from build123d import *

# Parameters (mm, degrees)
SKETCH1_W            = 208
SKETCH1_H            = 147
BOSS_EXTRUDE1_DEPTH  = 1
CUT_EXTRUDE1_DEPTH   = 128.354819304
MIRROR2_COPY_1_DEPTH = 128.354819304
FILLET1_R            = 10
CUT_EXTRUDE2_DEPTH   = 128.354819304
BOSS_EXTRUDE2_DEPTH  = 20
FILLET2_R            = 5
FILLET2_OF_MIRROR3_R = 5
MIRROR4_START        = 1
MIRROR4_DEPTH        = 20
SKETCH7_R            = 4
BOSS_EXTRUDE3_DEPTH  = 45
SKETCH8_R            = 3
CUT_EXTRUDE4_DEPTH   = 30


# Read off the part's stored shape, not the designer's step: Mirror4
with BuildPart() as part:
    # Sketch1 → Boss-Extrude1 (new body)
    with BuildSketch(Plane(origin=(0, 0, 0), x_dir=(1, 0, 0), z_dir=(0, 1, 0))):
        Rectangle(SKETCH1_W, SKETCH1_H)
    extrude(amount=BOSS_EXTRUDE1_DEPTH)

    # Sketch3 → Cut-Extrude1 (cut, through all)
    with BuildSketch(Plane(origin=(0, 1, 0), x_dir=(1, 0, 0), z_dir=(0, 1, 0))):
        with BuildLine():
            Line((-89, 83.145473262), (-89, 63.145473262))
            Line((-89, 63.145473262), (-44, 63.145473262))
            Line((-44, 63.145473262), (-44, 58.145473262))
            Line((-44, 58.145473262), (-29, 58.145473262))
            Line((-29, 58.145473262), (-29, 63.145473262))
            Line((-29, 63.145473262), (-14, 63.145473262))
            ThreePointArc((-14, 63.145473262), (-6.928932188, 63.647998579), (0, 65.145473262))
            Line((0, 65.145473262), (0, 85.145473262))
            Line((0, 85.145473262), (-89, 85.145473262))
            Line((-89, 85.145473262), (-89, 83.145473262))
        make_face()
    cut_extrude1 = extrude(amount=-CUT_EXTRUDE1_DEPTH, mode=Mode.SUBTRACT)

    # Mirror1: Cut-Extrude1 across plane
    add(cut_extrude1.mirror(Plane.XY), mode=Mode.SUBTRACT)

    # Mirror2: Cut-Extrude1 across plane
    add(cut_extrude1.mirror(Plane(origin=(0, 0, 0), x_dir=(0, 0, 1), z_dir=(1, 0, 0))), mode=Mode.SUBTRACT)

    # Mirror2 copy 1 sketch → Mirror2 copy 1 (cut, through all)
    with BuildSketch(Plane(origin=(0, 1, 0), x_dir=(-1, 0, 0), z_dir=(0, 1, 0))):
        with BuildLine():
            Line((-89, 83.145473262), (-89, 63.145473262))
            Line((-89, 63.145473262), (-44, 63.145473262))
            Line((-44, 63.145473262), (-44, 58.145473262))
            Line((-44, 58.145473262), (-29, 58.145473262))
            Line((-29, 58.145473262), (-29, 63.145473262))
            Line((-29, 63.145473262), (-14, 63.145473262))
            ThreePointArc((-14, 63.145473262), (-6.928932188, 63.647998579), (0, 65.145473262))
            Line((0, 65.145473262), (0, 85.145473262))
            Line((0, 85.145473262), (-89, 85.145473262))
            Line((-89, 85.145473262), (-89, 83.145473262))
        make_face()
    extrude(amount=-MIRROR2_COPY_1_DEPTH, mode=Mode.SUBTRACT)

    # Fillet1
    fillet1_edges = [part.edges().sort_by_distance(p)[0] for p in [
        (104, 0.5, 73.5),
        (-104, 0.5, 73.5),
        (-104, 0.5, -73.5),
        (104, 0.5, -73.5),
    ]]
    fillet(fillet1_edges, radius=FILLET1_R)

    # Sketch4 → Cut-Extrude2 (cut, through all)
    with BuildSketch(Plane.XZ):
        with BuildLine():
            Line((-58.225796132, 1.876244538), (-49.924870206, 1.876244538))
            ThreePointArc((-49.924870206, 1.876244538), (-49.217763425, 1.583351319), (-48.924870206, 0.876244538))
            Line((-48.924870206, 0.876244538), (-48.924870206, -0.876244538))
            ThreePointArc((-48.924870206, -0.876244538), (-49.217763425, -1.583351319), (-49.924870206, -1.876244538))
            Line((-49.924870206, -1.876244538), (-58.225796132, -1.876244538))
            ThreePointArc((-58.225796132, -1.876244538), (-58.932902913, -2.169137757), (-59.225796132, -2.876244538))
            Line((-59.225796132, -2.876244538), (-59.225796132, -11.176244538))
            ThreePointArc((-59.225796132, -11.176244538), (-59.518689351, -11.883351319), (-60.225796132, -12.176244538))
            Line((-60.225796132, -12.176244538), (-62.62394428, -12.176244538))
            ThreePointArc((-62.62394428, -12.176244538), (-63.331051061, -11.883351319), (-63.62394428, -11.176244538))
            Line((-63.62394428, -11.176244538), (-63.62394428, -2.876244538))
            ThreePointArc((-63.62394428, -2.876244538), (-63.916837499, -2.169137757), (-64.62394428, -1.876244538))
            Line((-64.62394428, -1.876244538), (-72.924870206, -1.876244538))
            ThreePointArc((-72.924870206, -1.876244538), (-73.631976987, -1.583351319), (-73.924870206, -0.876244538))
            Line((-73.924870206, -0.876244538), (-73.924870206, 0.876244538))
            ThreePointArc((-73.924870206, 0.876244538), (-73.631976987, 1.583351319), (-72.924870206, 1.876244538))
            Line((-72.924870206, 1.876244538), (-64.62394428, 1.876244538))
            ThreePointArc((-64.62394428, 1.876244538), (-63.916837499, 2.169137757), (-63.62394428, 2.876244538))
            Line((-63.62394428, 2.876244538), (-63.62394428, 11.823755462))
            ThreePointArc((-63.62394428, 11.823755462), (-63.331051061, 12.530862243), (-62.62394428, 12.823755462))
            Line((-62.62394428, 12.823755462), (-60.225796132, 12.823755462))
            ThreePointArc((-60.225796132, 12.823755462), (-59.518689351, 12.530862243), (-59.225796132, 11.823755462))
            Line((-59.225796132, 11.823755462), (-59.225796132, 2.876244538))
            ThreePointArc((-59.225796132, 2.876244538), (-58.932902913, 2.169137757), (-58.225796132, 1.876244538))
        make_face()
    extrude(amount=-CUT_EXTRUDE2_DEPTH, mode=Mode.SUBTRACT)

    # Sketch5 → Boss-Extrude2 (add)
    with BuildSketch(Plane(origin=(0, 1, 0), x_dir=(1, 0, 0), z_dir=(0, 1, 0))):
        Polygon((-104, 36.429300806), (-11, 36.429300806), (-11, 63.235554408), (-14, 63.145473262), (-14, 39.429300806), (-104, 39.429300806), align=None)
    boss_extrude2 = extrude(amount=BOSS_EXTRUDE2_DEPTH)

    # Fillet2
    fillet2_edges = [part.edges().sort_by_distance(p)[0] for p in [
        (-11, 11, -36.429300806),
    ]]
    fillet(fillet2_edges, radius=FILLET2_R)

    # Mirror3: Boss-Extrude2 across plane
    add(boss_extrude2.mirror(Plane.XY))

    # Fillet2 of Mirror3
    fillet2_of_mirror3_edges = [part.edges().sort_by_distance(p)[0] for p in [
        (-11, 11, 36.429300806),
    ]]
    fillet(fillet2_of_mirror3_edges, radius=FILLET2_OF_MIRROR3_R)

    # Mirror4 outline → Mirror4 (add)
    with BuildSketch(Plane(origin=(0, 0, 0), x_dir=(1, 0, 0), z_dir=(0, 1, 0)).offset(MIRROR4_START)):
        with BuildLine():
            Line((104, -39.429300806), (104, -36.429300806))
            Line((104, -36.429300806), (16, -36.429300806))
            ThreePointArc((16, -36.429300806), (12.464466094, -37.8937669), (11, -41.429300806))
            Line((11, -41.429300806), (11, -63.235554408))
            Line((11, -63.235554408), (14, -63.145473262))
            Line((14, -63.145473262), (14, -39.429300806))
            Line((14, -39.429300806), (104, -39.429300806))
        make_face()
        with BuildLine():
            Line((104, 36.429300806), (104, 39.429300806))
            Line((104, 39.429300806), (14, 39.429300806))
            Line((14, 39.429300806), (14, 63.145473262))
            Line((14, 63.145473262), (11, 63.235554408))
            Line((11, 63.235554408), (11, 41.429300806))
            ThreePointArc((11, 41.429300806), (12.464466094, 37.8937669), (16, 36.429300806))
            Line((16, 36.429300806), (104, 36.429300806))
        make_face()
    extrude(amount=MIRROR4_DEPTH)

    # Sketch7 → Boss-Extrude3 (add)
    with BuildSketch(Plane.XZ):
        with Locations(Location((97, 65, 0), (0, 0, 90))):
            Circle(SKETCH7_R)
        with Locations(Location((-95, 65, 0), (0, 0, 90))):
            Circle(SKETCH7_R)
        with Locations(Location((-95, -65, 0), (0, 0, 90))):
            Circle(SKETCH7_R)
        with Locations(Location((97, -65, 0), (0, 0, 90))):
            Circle(SKETCH7_R)
    extrude(amount=BOSS_EXTRUDE3_DEPTH)

    # Sketch8 → Cut-Extrude4 (cut)
    with BuildSketch(Plane(origin=(0, -45, 0), x_dir=(-1, 0, 0), z_dir=(0, -1, 0))):
        with Locations(Location((95, 65, 0), (0, 0, 90))):
            Circle(SKETCH8_R)
        with Locations(Location((95, -65, 0), (0, 0, 90))):
            Circle(SKETCH8_R)
        with Locations(Location((-97, -65, 0), (0, 0, 90))):
            Circle(SKETCH8_R)
        with Locations(Location((-97, 65, 0), (0, 0, 90))):
            Circle(SKETCH8_R)
    extrude(amount=-CUT_EXTRUDE4_DEPTH, mode=Mode.SUBTRACT)


solid = part.part
Could you check a few things on this model? Use its own coordinates, in mm. A direction names the side the tool comes from. Coordinates: 2 decimals unless noted, no trailing zeros. Order: outer loops, then holes, each group sorted by start corner. A loop starts at its lowest first (then second) coordinate and runs counter-clockwise, first axis right, second up. Notation, with made-up numbers: (70.25, 26.5) -> (82.25, 26.5) arc R15 cw to (82.25, 36.5) -> close; hole circle Ø9 at (-7, 54.25). An arc over 180 degrees is marked (long way). One line per item, written item: value. Start each with the question number.
1) We'd pull the mould along Z, two halves only. Please class faces 1 (the flat face through (58, 1, 52)), 2 (the cylindrical face through (101.15, 0.51, 70.49)), 3 (the flat face through (-95, -15, -65)): +Z half, -Z half, draft (parallel to the pull), parting line (faces both ways), or undercut.
2) Imagine slicing it at B-B on z = -9. List the corners of the cut face in (x, y) for me, plus the area to 3 significant figures.
3) If I drill on L1, parallel to X at y = -31, z = -65; L2, parallel to Z at x = 40, y = 17; L3, parallel to Y at x = -50, z = 53, over which ranges is the centre line in solid material (lowest first)? Write a range as [from, to].
4) Imagine slicing it at D-D on x = 57. List the corners of the cut face in (y, z) for me, plus the area to 3 significant figures.
5) Which directions (+Z, -Z, +X, -X, +Y, -Y) give clear straight access to the entire face, cutting with the end or side of a thin tool? Please do faces 4 (the flat face through (-60, 1, 52)), 5 (the flat face through (-58, 11, -39.429)), 6 (the cylindrical face through (94.07, -30.21, -64.35)), 7 (the flat face through (-11, 11, -52)).
6) Imagine slicing it at A-A on y = -19.5. List the corners of the cut face in (x, z) for me, plus the area to 3 significant figures.
7) I'm going to push flat-ended pins straight in: pin 1 (3.5 mm diameter, centred on x = -95, z = 65, fed in from +Y); pin 2 (6 mm diameter, centred on x = 4.5, z = 18, fed in from -Y); pin 3 (1.1 mm diameter, centred on x = 22.5, y = 0.5, fed in from -Z). Where does each tip first touch, or does it pass through?
8) Imagine slicing it at C-C on y = 15. List the corners of the cut face in (x, z) for me, plus the area to 3 significant figures.
Answer list:
1. face 1: draft
1. face 2: +Z half
1. face 3: undercut
2. outline: (-104, 0) -> (-63.62, 0) -> (-63.62, 1) -> (-104, 1) -> close; (-59.23, 0) -> (104, 0) -> (104, 1) -> (-59.23, 1) -> close
2. area: 204 mm2
3. L1: x = [-99, -98], [-92, -91], [93, 94], [100, 101]
3. L2: z = [-39.43, -36.43], [36.43, 39.43]
3. L3: y = [0, 1]
4. outline: (0, -63.15) -> (1, -63.15) -> (1, -39.43) -> (21, -39.43) -> (21, -36.43) -> (1, -36.43) -> (1, 36.43) -> (21, 36.43) -> (21, 39.43) -> (1, 39.43) -> (1, 63.15) -> (0, 63.15) -> close
4. area: 246 mm2
5. face 4: +Z, -X, +Y
5. face 5: -Z, -X, +Y
5. face 6: -Y
5. face 7: +Z, -Z, +Y
6. outline: circle Ø8 at (-95, -65); circle Ø8 at (-95, 65); circle Ø8 at (97, -65); circle Ø8 at (97, 65); hole circle Ø6 at (-95, -65); hole circle Ø6 at (-95, 65); hole circle Ø6 at (97, -65); hole circle Ø6 at (97, 65)
6. area: 88.0 mm2
7. pin 1: stops at y = 1
7. pin 2: stops at y = 0
7. pin 3: stops at z = -63.15
8. outline: (-104, -39.43) -> (-14, -39.43) -> (-14, -63.15) -> (-11, -63.24) -> (-11, -41.43) arc R5 ccw to (-16, -36.43) -> (-104, -36.43) -> close; (-104, 36.43) -> (-16, 36.43) arc R5 ccw to (-11, 41.43) -> (-11, 63.24) -> (-14, 63.15) -> (-14, 39.43) -> (-104, 39.43) -> close; (11, -63.24) -> (14, -63.15) -> (14, -39.43) -> (104, -39.43) -> (104, -36.43) -> (16, -36.43) arc R5 ccw to (11, -41.43) -> close; (11, 41.43) arc R5 ccw to (16, 36.43) -> (104, 36.43) -> (104, 39.43) -> (14, 39.43) -> (14, 63.15) -> (11, 63.24) -> close
8. area: 1,380 mm2
